Here's the drawing with two shaded views (mm, measured from the low corner). I have some questions. Coordinates: 2 decimals unless noted, no trailing zeros. Answer as CSV lines item,"result". Start each with the question number.
1. I want a section at A-A, the plane y = 91.5. Count the separate pieces of the cut face and the enclosed holes in it.
2. Thinking about a two-plate mould opening in Z: for the marked faces 1 and 2, which applies, released by +Z, released by -Z, zero draft, split by the parting line, or undercut?
3. I need wall thicknesses on probe 1 along X at (y, z) = (14.5, 2.7). Which ranges of the line are inside material? Lowest first, please.
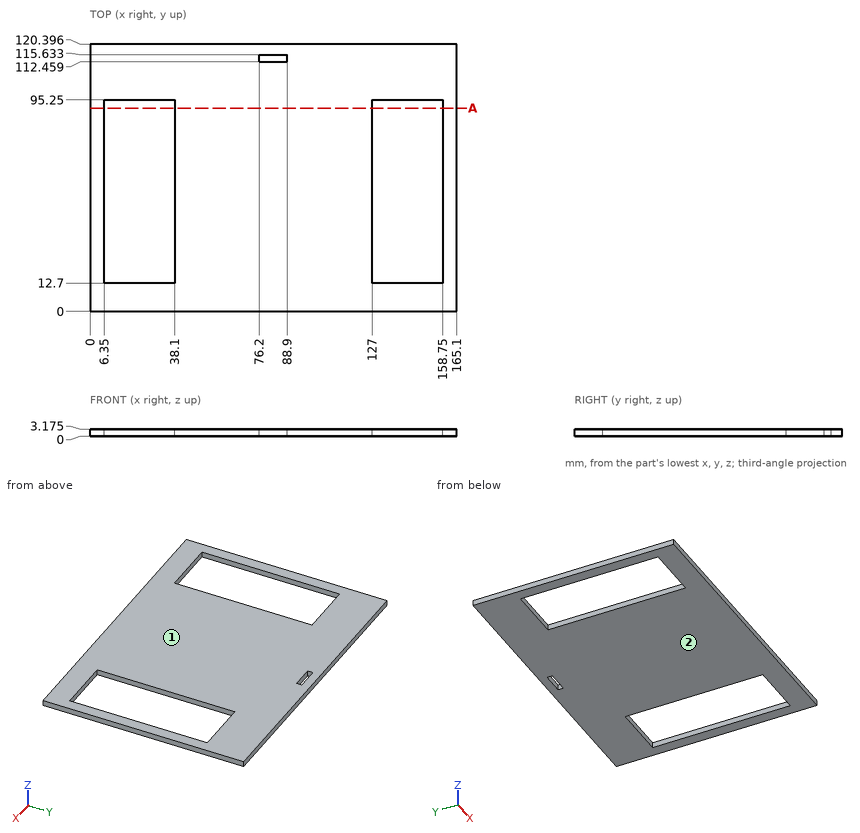
Solved:
1,separate pieces,"3"
1,enclosed holes,"0"
2,face 1,"released by +Z"
2,face 2,"released by -Z"
3,probe 1,"x = 0 to 6.35, 38.1 to 127, 158.75 to 165.1"
